```python
from build123d import *

# Parameters (mm, degrees)
FILLET1_R   = 0.4
HEX_2_DEPTH = 2.6


with BuildPart() as part:
    # BodySke → BaseBody (revolve)
    with BuildSketch(Plane.XY, mode=Mode.PRIVATE) as basebody_sk:
        with BuildLine():
            Line((34.4, 0), (34.4, 3.3095))
            Line((34.4, 3.3095), (33.7095, 4))
            Line((33.7095, 4), (4.4, 4))
            Line((4.4, 4), (4.4, 7))
            Line((4.4, 7), (4.02, 7))
            ThreePointArc((4.02, 7), (1.686451133, 5.621618984), (0, 3.5))
            Line((0, 3.5), (0, 0))
            Line((0, 0), (34.4, 0))
        make_face()
    revolve(basebody_sk.sketch.rotate(Axis((0, 0, 0), (1, 0, 0)), 90), axis=Axis((0, 0, 0), (1, 0, 0)))  # turned: the seam where the file's is

    # Fillet1
    fillet1_edges = [part.edges().sort_by_distance(p)[0] for p in [
        (4.4, 0, -4),
    ]]
    fillet(fillet1_edges, radius=FILLET1_R)

    # Sketch2 → PreBroach (revolve, cut)
    with BuildSketch(Plane.XY, mode=Mode.PRIVATE) as prebroach_sk:
        Polygon((0, 2.5), (2.6, 2.5), (4.043375673, 0), (0, 0), align=None)
    revolve(prebroach_sk.sketch.rotate(Axis((0, 0, 0), (1, 0, 0)), 90), axis=Axis((0, 0, 0), (1, 0, 0)), mode=Mode.SUBTRACT)  # turned: the seam where the file's is

    # Sketch3 → Hex 2 (cut)
    with BuildSketch(Plane(origin=(0, 0, 0), x_dir=(0, 0, -1), z_dir=(1, 0, 0))):
        Polygon((-2.5, -1.443375673), (-2.5, 1.443375673), (0, 2.886751346), (2.5, 1.443375673), (2.5, -1.443375673), (0, -2.886751346), align=None)
    extrude(amount=HEX_2_DEPTH, mode=Mode.SUBTRACT)


solid = part.part
```
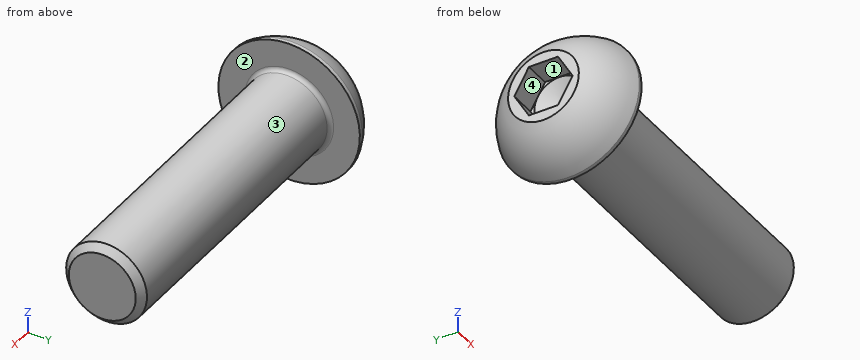
Could you check a few things on this model? Use its own coordinates, in mm. Face numbers are marked on the shaded views. Give positions to 0.01 mm unless a question says otherwise; leave off trailing zeros. Write each loop counter-clockwise with the first axis right and the second up, starting at its lowest first coordinate (ties: lowest second). Pieces come first, ordered by that corner, then holes. Notation, with made-up numbers: (-4, 17) - (35, 17) arc R30 ccw to (35, 50) - close; hole circle Ø11 at (72.25, 51.25). An arc over 180 degrees is marked (long way). One line per item, written item: value. Start each with the question number.
Item 1: If we mould it in two halves opening along Y, with no side actions, what happens to the marked faces 1, 2, 3 and 4? For each: +Y half, -Y half, draft (parallel to the pull), parting line (faces both ways), or undercut.
Item 2: I'm going to push flat-ended pins straight in: pin 1 (1.4 mm diameter, centred on y = 0.5, z = -1.5, fed in from -X); pin 2 (1.5 mm diameter, centred on x = 30, z = -1.5, fed in from +Y); pin 3 (2 mm diameter, centred on x = 21.5, y = 4.5, fed in from +Z); pin 4 (1 mm diameter, centred on x = 9, z = -5, fed in from +Y). Where does each tip first touch, or does it pass through?
Item 3: Imagine slicing it at C-C, the plane y = -5. List the corners of the cut face in (x, z) for me.
Item 4: Imagine slicing it at A-A, the plane x = 26.5. List the corners of the cut face in (y, z) for me, and give its area (3 significant figures).
Item 5: Imagine slicing it at B-B, the plane y = 6.25. List the corners of the cut face in (x, z) for me, and give its area (3 significant figures).
Item 6: Please list where these lines run through material, in increasing order: line 1 (Y direction, x = 16.5, z = 2.25); line 2 (X direction, y = -6, z = 2.75). Write a range as from..to.
Geometry says:
1. face 1: undercut
1. face 2: draft
1. face 3: parting line
1. face 4: undercut
2. pin 1: x = 2.73
2. pin 2: y = 3.93
2. pin 3: z = 1.94
2. pin 4: through
3. outline: (4.02, -4.9) - (4.4, -4.9) - (4.4, 4.9) - (4.02, 4.9) arc R5.53 ccw to start
4. outline: circle Ø8 at (0, 0)
4. area: 50.3 mm^2
5. outline: (4.02, -3.15) - (4.4, -3.15) - (4.4, 3.15) - (4.02, 3.15) arc R4.06 ccw to start
5. area: 8.98 mm^2
6. line 1: -3.31..3.31
6. line 2: 3.12..4.4
